Part model, mm, in its own coordinate system. A direction names the side the tool comes from. Round coordinates to 2 decimals unless told otherwise and drop trailing zeros. Order: outer loops, then holes, each group sorted by start corner. A loop starts at its lowest first (then second) coordinate and runs counter-clockwise, first axis right, second up. Notation, with made-up numbers: (-6, -26) - (13, -26) arc R19 cw to (13, -13) - close; hole circle Ø7 at (8.5, -7). An arc over 180 degrees is marked (long way). Answer as a JSON object with one key per item and string values.
```python
from build123d import *
from build123d.topology import SkipClean

# Parameters (mm, degrees)
SKETCH_1_W           = 20
SKETCH_1_H           = 50
EXTRUDE_2_DEPTH      = 20
SKETCH_2_W           = 20
SKETCH_2_H           = 10
CUT_EXTRUDE_1_DEPTH  = 20
CUT_EXTRUDE_2_DEPTH  = 20
CUT_EXTRUDE_3_DEPTH  = 20
CUT_EXTRUDE_4_DEPTH  = 20
SKETCH_6_W           = 13
SKETCH_6_H           = 13
CUT_EXTRUDE_5_DEPTH  = 25
EXTRUDE_3_DEPTH      = 8
EXTRUDE_6_DEPTH      = 10
EXTRUDE_6_DEPTH_BACK = 20
CUT_EXTRUDE_7_DEPTH  = 18
CUT_EXTRUDE_8_DEPTH  = 26
CUT_EXTRUDE_9_DEPTH  = 26


with BuildPart() as part:
    # 草图1 → 凸台-拉伸2 (new body)
    with BuildSketch(Plane(origin=(0, 0, 0), x_dir=(0, 0, -1), z_dir=(1, 0, 0))):
        Rectangle(SKETCH_1_W, SKETCH_1_H)
    extrude(amount=EXTRUDE_2_DEPTH)

    # 草图2 → 切除-拉伸1 (cut)
    with BuildSketch(Plane(origin=(20, 0, 0), x_dir=(0, 0, -1), z_dir=(1, 0, 0))):
        with Locations((0, -20)):
            Rectangle(SKETCH_2_W, SKETCH_2_H)
    extrude(amount=-CUT_EXTRUDE_1_DEPTH, mode=Mode.SUBTRACT)

    # 草图3 → 切除-拉伸2 (cut)
    with BuildSketch(Plane(origin=(0, 0, -10), x_dir=(-1, 0, 0), z_dir=(0, 0, -1))):
        with BuildLine():
            Line((-15, 21.75), (-5, 21.75))
            ThreePointArc((-5, 21.75), (-2.25, 19), (-5, 16.25))
            Line((-5, 16.25), (-15, 16.25))
            ThreePointArc((-15, 16.25), (-17.75, 19), (-15, 21.75))
        make_face()
    extrude(amount=-CUT_EXTRUDE_2_DEPTH, mode=Mode.SUBTRACT)

    # 草图4 → 切除-拉伸3 (cut)
    with BuildSketch(Plane.ZY):
        with BuildLine():
            Line((-5, 11.5), (5, 11.5))
            ThreePointArc((5, 11.5), (7.5, 9), (5, 6.5))
            Line((5, 6.5), (-5, 6.5))
            ThreePointArc((-5, 6.5), (-7.5, 9), (-5, 11.5))
        make_face()
    extrude(amount=-CUT_EXTRUDE_3_DEPTH, mode=Mode.SUBTRACT)

    # 草图5 → 切除-拉伸4 (cut)
    with BuildSketch(Plane(origin=(0, 0, -10), x_dir=(-1, 0, 0), z_dir=(0, 0, -1))):
        with BuildLine():
            Line((-15, 2.75), (-5, 2.75))
            ThreePointArc((-5, 2.75), (-2.25, 0), (-5, -2.75))
            Line((-5, -2.75), (-15, -2.75))
            ThreePointArc((-15, -2.75), (-17.75, 0), (-15, 2.75))
        make_face()
    extrude(amount=-CUT_EXTRUDE_4_DEPTH, mode=Mode.SUBTRACT)

    # 草图6 → 切除-拉伸5 (cut)
    with BuildSketch(Plane.XZ.offset(15)):
        with Locations((6.5, 3.5)):
            Rectangle(SKETCH_6_W, SKETCH_6_H)
    extrude(amount=-CUT_EXTRUDE_5_DEPTH, mode=Mode.SUBTRACT)

    # 草图7 → 凸台-拉伸3 (add)
    with BuildSketch(Plane(origin=(0, 25, 0), x_dir=(1, 0, 0), z_dir=(0, 1, 0))):
        Polygon((-16.213203436, -16.213203436), (-6.213203436, -26.213203436), (10, -10), (0, 0), align=None)
    extrude(amount=-EXTRUDE_3_DEPTH)

    # 草图8 → 凸台-拉伸6 (add, two sides: drawn at the far end of the back side and taken through both)
    with BuildSketch(Plane(origin=(0, 0, 0), x_dir=(-0.707106781186539, 0, 0.707106781186556), z_dir=(-0.707106781186556, 0, -0.707106781186539)).offset(-EXTRUDE_6_DEPTH_BACK)):
        Polygon((18.197319143, 27), (34.979311766, 7), (37.590126345, 7), (20.808133721, 27), align=None)
    extrude(amount=EXTRUDE_6_DEPTH + EXTRUDE_6_DEPTH_BACK)

    # 草图11 → 切除-拉伸7 (cut)
    with BuildSketch(Plane(origin=(10, 0, 10), x_dir=(0.7071067811865497, 0, -0.7071067811865454), z_dir=(0.7071067811865454, 0, 0.7071067811865497))):
        Polygon((-22.928932188, 24.472530808), (-22.486332984, 25), (-22.928932188, 25), align=None)
    extrude(amount=-CUT_EXTRUDE_7_DEPTH, mode=Mode.SUBTRACT)

    # 草图12 → 切除-拉伸8 (cut)
    with SkipClean():  # the faces are left unmerged after this step: merging them gives an invalid solid
        with BuildSketch(Plane(origin=(0, 0, -10), x_dir=(-1, 0, 0), z_dir=(0, 0, -1))):
            with BuildLine():
                Line((-15, 16.25), (-5, 16.25))
                ThreePointArc((-5, 16.25), (-2.25, 19), (-5, 21.75))
                Line((-5, 21.75), (-15, 21.75))
                ThreePointArc((-15, 21.75), (-17.75, 19), (-15, 16.25))
            make_face()
        extrude(amount=-CUT_EXTRUDE_8_DEPTH, mode=Mode.SUBTRACT)
    add(part.part.scale(1), mode=Mode.REPLACE)  # the faces are merged on a copy

    # 草图13 → 切除-拉伸9 (cut)
    with BuildSketch(Plane(origin=(0, 25, 0), x_dir=(1, 0, 0), z_dir=(0, 1, 0))):
        with BuildLine():
            Line((-9.534541797, -16.138807841), (1.572830507, -5.47197893))
            ThreePointArc((1.572830507, -5.47197893), (4.614784317, -5.533524822), (4.553238425, -8.575478633))
            Line((4.553238425, -8.575478633), (-6.554133879, -19.242307544))
            ThreePointArc((-6.554133879, -19.242307544), (-9.596087689, -19.180761651), (-9.534541797, -16.138807841))
        make_face()
    extrude(amount=-CUT_EXTRUDE_9_DEPTH, mode=Mode.SUBTRACT)


solid = part.part
```
Item 1: Cut at C-C (z = 21.5). Write the cut outline in (x, y), plus the area to 3 significant figures.
Taken from the geometry:
{"outline": "(-31.66, 7) - (-27.97, 7) - (-10.93, 21.36) - (-10.93, 17) - (-1.5, 17) - (-1.5, 25) - (-6.61, 25) - (-4.23, 27) - (-7.93, 27) - close", "area": "141 mm2"}
Item 2: Tool access for faces 1 (the flat face through (0, 21, 20)), 2 (the flat face through (6, -4, -3)), 3 (the flat face through (10, 11.5, 0)), 4 (the cylindrical face through (17.75, 18.94, -0.14)), 5 (the flat face through (-4.06, 21.08, 10.88)): list every direction of +Z, -Z, +X, -X, +Y, -Y with a clear straight run to the whole face (end or side of a thin tool).
Taken from the geometry:
{"face 1": "+X, -Y", "face 2": "+Z, -X, -Y", "face 3": "+X, -X", "face 4": "+Z, -Z", "face 5": "+Y, -Y"}
Item 3: Cut at A-A (y = 0). Write the cut outline in (x, z).
Taken from the geometry:
{"outline": "(0, -10) - (2.25, -10) - (2.25, -3) - (0, -3) - close; (17.75, -10) - (20, -10) - (20, 10) - (17.75, 10) - close"}
Item 4: Probe L1, parallel to X at y = 19, z = 0; L2, parallel to X at y = 21, z = 15.5; L3, parallel to Y at x = 10.5, z = 0. List the from-to ranges inside material, lowest first. Write a range as from..to.
Taken from the geometry:
{"L1": "0..2.25, 17.75..20", "L2": "-21.05..-17.35, -15.5..-8.87, -2.66..3.11", "L3": "11.5..16.25, 21.75..25"}
Item 5: Cut at D-D (y = 23). Write the cut outline in (x, z), plus the area to 3 significant figures.
Taken from the geometry:
{"outline": "(-24.16, 10.02) - (-22.31, 8.17) - (-15.24, 15.24) - (0, 0) - (0, -10) - (20, -10) - (20, 10) - (10, 10) - (-5.24, 25.24) - (-1.1, 29.38) - (-2.94, 31.23) - close; hole (-9.53, 16.14) - (1.57, 5.47) arc R2.15 ccw to (4.55, 8.58) - (-6.55, 19.24) arc R2.15 ccw to start", "area": "652 mm2"}
Item 6: Cut at B-B (y = 5). Write the cut outline in (x, z).
Taken from the geometry:
{"outline": "(0, -10) - (20, -10) - (20, 10) - (13, 10) - (13, -3) - (0, -3) - close"}
Item 7: Two-plate mould, pull along Y, no slides. Class faces 6 (the flat face through (-8, 21, 8)), 7 (the flat face through (11, 2.75, -5)), 8 (the flat face through (-9.4, 25, 19)): pulls with the +Y half, pulls with the -Y half, needs draft (parallel to the pull), parting line crosses it, or undercut.
Taken from the geometry:
{"face 6": "needs draft", "face 7": "undercut", "face 8": "pulls with the -Y half"}
Item 8: Drop flat-ended pins along their axis: P1, Ø6.5, axis at x = 6, y = -6, coming from the +Z side; P2, Ø4, axis at y = 8.5, z = 8, coming from the -X side (3 decimals); P3, Ø3.5, axis at y = 6, z = 2.5, coming from the -X side. Give the stop position or say it passes through.
Taken from the geometry:
{"P1": "z = -3", "P2": "x = 3.775", "P3": "x = 13"}
